Answer from the drawing. Dimensions are ordinates in mm from the lowest x, y and z of the part. A direction names the side the tool comes from. Give positions to 0.01 mm unless a question says otherwise; leave off trailing zeros. Order: outer loops, then holes, each group sorted by start corner. A loop starts at its lowest first (then second) coordinate and runs counter-clockwise, first axis right, second up. Notation, with made-up numbers: (42.25, 5.25) - (74.25, 5.25) arc R21 ccw to (74.25, 17.25) - close; hole circle Ø3 at (59.25, 85). An arc over 180 degrees is marked (long way). Answer in a Markdown table with one row per item. Add a question column.
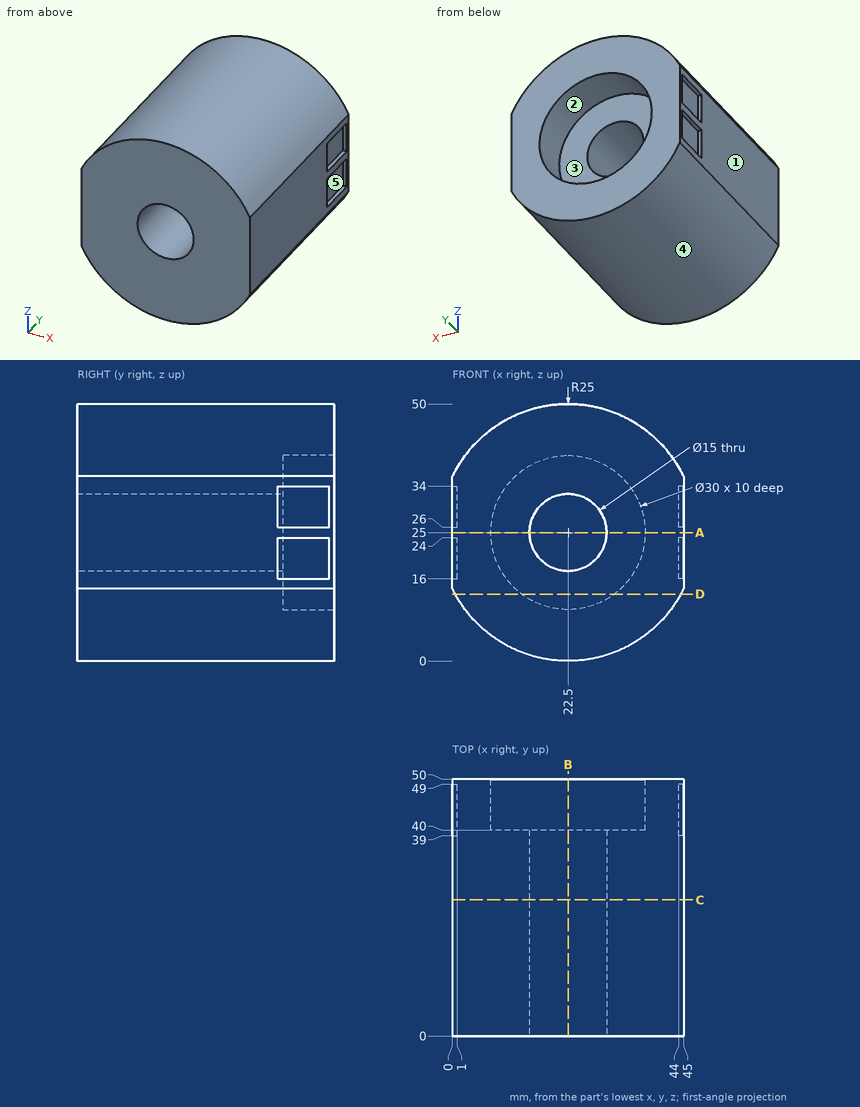
(1) Find section D-D, the plane z = 13. Write down the section's boundary in (x, y), plus the area to 3 significant figures.
(2) Find section B-B, the plane x = 22.5. Write down the section's boundary in (y, z).
(3) For the marked faces 1 and 2, determine the directions among +Z, -Z, +X, -X, +Y, -Y from which every point of the face is accessible in a straight line to the end or side of a thin tool.
(4) Find section A-A, the plane z = 25. Write down the section's boundary in (x, y), plus the area to 3 significant figures.
(5) The mould has two halves that part along Y. Classify the marked faces 3, 4 and 5: +Y half, -Y half, draft (parallel to the pull), parting line (faces both ways), or undercut.
(6) Each of these flat-tipped pins is pushed along its axis until it touches: P1, Ø4, axis at y = 44.5, z = 31, coming from the +X side; P2, Ø6, axis at x = 5, y = 12.5, coming from the -Z side; P3, Ø0.5, axis at x = 0.5, y = 46.5, coming from the -Z side. Where does it stop, or does it pass through?
(7) Straight lines are drawn through the part: line 1 (X direction, y = 19.5, z = 25); line 2 (Z direction, x = 22, y = 44) (3 decimals); line 3 (X direction, y = 46, z = 25). For each, find the intervals that lie inside material, in ascending order.
(8) Find section C-C, the plane y = 26.5. Write down the section's boundary in (x, z).
Answer key:
| question | item | result |
|---|---|---|
| 1 | outline | (0.57, 0) - (44.43, 0) - (44.43, 50) - (31.5, 50) - (31.5, 40) - (13.5, 40) - (13.5, 50) - (0.57, 50) - close |
| 1 | area | 2,010 mm² |
| 2 | outline | (0, 0) - (50, 0) - (50, 10) - (40, 10) - (40, 17.5) - (0, 17.5) - close; (0, 32.5) - (40, 32.5) - (40, 40) - (50, 40) - (50, 50) - (0, 50) - close |
| 3 | face 1 | +Z, -Z, -X, +Y, -Y |
| 3 | face 2 | +Y |
| 4 | outline | (0, 0) - (15, 0) - (15, 40) - (7.5, 40) - (7.5, 50) - (0, 50) - close; (30, 0) - (45, 0) - (45, 50) - (37.5, 50) - (37.5, 40) - (30, 40) - close |
| 4 | area | 1,350 mm² |
| 5 | face 3 | +Y half |
| 5 | face 4 | draft |
| 5 | face 5 | undercut |
| 6 | P1 | x = 44 |
| 6 | P2 | z = 4.63 |
| 6 | P3 | z = 12.67 |
| 7 | line 1 | 0 to 15, 30 to 45 |
| 7 | line 2 | 0.005 to 10.008, 39.992 to 49.995 |
| 7 | line 3 | 0 to 7.5, 37.5 to 45 |
| 8 | outline | (0, 14.1) arc R25 ccw to (45, 14.1) - (45, 35.9) arc R25 ccw to (0, 35.9) - close; hole circle Ø15 at (22.5, 25) |
